Design review of the part built by this model. Coordinates are the model's own, in mm. Face numbers are marked on the shaded views. Coordinates: 2 decimals unless noted, no trailing zeros. Order: outer loops, then holes, each group sorted by start corner. A loop starts at its lowest first (then second) coordinate and runs counter-clockwise, first axis right, second up. Notation, with made-up numbers: M 86,56.5 L 135,56.5 A24 ccw 135,76.5 Z; hole C 1,6 d6. An arc over 180 degrees is marked long. Use CSV: the item, a comma, the result in double quotes.
```python
from build123d import *

# Parameters (mm, degrees)
SKETCH_3_R               = 40
EXTRUDE_2_DEPTH          = 5
CUT_EXTRUDE_2_DEPTH      = 10
SKETCH_6_R               = 2
CUT_EXTRUDE_3_DEPTH      = 10
SKETCH_8_R               = 3.5
SKETCH_8_R_2             = 2.5
EXTRUDE_3_DEPTH          = 8
PATTERN_CIRCULAR_1_COUNT = 3


with BuildPart() as part:
    # 草图3 → 凸台-拉伸2 (new body)
    with BuildSketch(Plane(origin=(0, 0, 0), x_dir=(1, 0, 0), z_dir=(0, 1, 0))):
        with Locations(Location((0, 0, 0), (0, 0, 270))):
            Circle(SKETCH_3_R)
    extrude(amount=EXTRUDE_2_DEPTH)

    # 草图5 → 切除-拉伸2 (cut)
    with BuildSketch(Plane(origin=(0, 5, 0), x_dir=(1, 0, 0), z_dir=(0, 1, 0))):
        with BuildLine():
            Line((-3, -29.849623113), (-3, 29.849623113))
            ThreePointArc((-3, 29.849623113), (-30, 0), (-3, -29.849623113))
        make_face()
        with BuildLine():
            ThreePointArc((30, 0), (22.248595461, 20.124611797), (3, 29.849623113))
            Line((3, 29.849623113), (3, -29.849623113))
            ThreePointArc((3, -29.849623113), (22.248595461, -20.124611797), (30, 0))
        make_face()
    extrude(amount=-CUT_EXTRUDE_2_DEPTH, mode=Mode.SUBTRACT)

    # 草图6 → 切除-拉伸3 (cut)
    with BuildSketch(Plane(origin=(0, 5, 0), x_dir=(1, 0, 0), z_dir=(0, 1, 0))):
        with Locations(Location((0, 0, 0), (0, 0, 270))):
            Circle(SKETCH_6_R)
    extrude(amount=-CUT_EXTRUDE_3_DEPTH, mode=Mode.SUBTRACT)

    # 草图8 → 凸台-拉伸3 (add)
    with BuildSketch(Plane(origin=(0, 5, 0), x_dir=(1, 0, 0), z_dir=(0, 1, 0))):
        with Locations(Location((0, -35, 0), (0, 0, 270))):
            Circle(SKETCH_8_R)
        with Locations(Location((0, -35, 0), (0, 0, 270))):
            Circle(SKETCH_8_R_2, mode=Mode.SUBTRACT)
    extrude_3 = extrude(amount=EXTRUDE_3_DEPTH)

    # 阵列(圆周)1: 凸台-拉伸3 ×3 about axis
    pattern_circular_1_axis = Axis((0, 0, 0), (0, 1, 0))
    for i in range(1, PATTERN_CIRCULAR_1_COUNT):
        add(extrude_3.rotate(pattern_circular_1_axis, i * 360 / PATTERN_CIRCULAR_1_COUNT))


solid = part.part
```
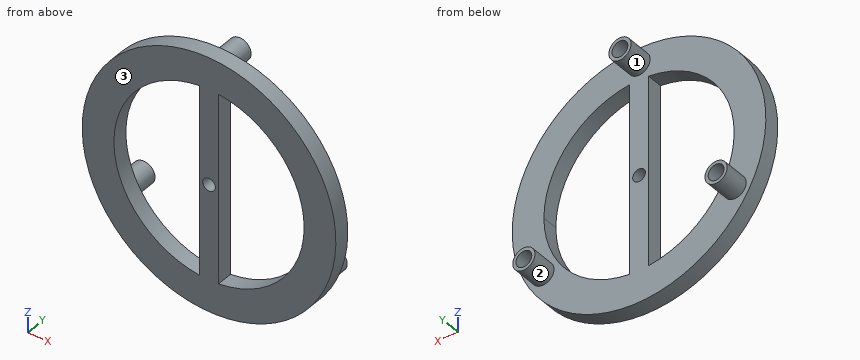
(1) Wall thickness on probe 1 along X at (y, z) = (1.65, 0); probe 2 along X at (y, z) = (11.25, -17.5); probe 3 along X at (y, z) = (3.5, -8.5): over which ranges is each line inside the solid? List them lowest first.
The answers:
probe 1,"x = -40 to -30, -3 to -2, 2 to 3, 30 to 40"
probe 2,"x = -33.81 to -32.81, -27.81 to -26.81, 26.81 to 27.81, 32.81 to 33.81"
probe 3,"x = -39.09 to -28.77, -3 to 3, 28.77 to 39.09"
(2) Clearance check with flat-ended pins moving along their axes: P1, Ø2.5, axis at y = 1.5, z = -9, coming from the +X side; P2, Ø2, axis at y = 4.5, z = -27.5, coming from the +X side; P3, Ø2.5, axis at x = -30, z = -18.5, coming from the +Y side; P4, Ø1.5, axis at x = 25, y = 6, coming from the -Z side. State where each tip first meets the part, or that it passes through.
The answers:
P1,"stops at x = 39.24"
P2,"stops at x = 29.96"
P3,"stops at y = 5"
P4,"passes through"
(3) Add section A-A on x = 0. State the section outline as (y, z) points, and give its area (3 significant figures).
The answers:
outline,"M 0,-40 L 5,-40 L 5,-2 L 0,-2 Z; M 0,2 L 5,2 L 5,31.5 L 13,31.5 L 13,32.5 L 5,32.5 L 5,37.5 L 13,37.5 L 13,38.5 L 5,38.5 L 5,40 L 0,40 Z"
area,"396 mm2"
(4) Add section D-D on y = 11.5. State the section outline as (x, z) points.
The answers:
outline,"C -30.31,-17.5 d7; C 0,35 d7; C 30.31,-17.5 d7; hole C -30.31,-17.5 d5; hole C 0,35 d5; hole C 30.31,-17.5 d5"
(5) Add section C-C on z = -3. State the section outline as (x, y) points, and give its area (3 significant figures).
The answers:
outline,"M -39.89,0 L -29.85,0 L -29.85,5 L -39.89,5 Z; M -3,0 L 3,0 L 3,5 L -3,5 Z; M 29.85,0 L 39.89,0 L 39.89,5 L 29.85,5 Z"
area,"130 mm2"
(6) The part is to be moulded in two halves that separate along X. For the marked faces 1, 2 and 3, say which applies: pulls with the +X half, pulls with the -X half, needs draft (parallel to the pull), parting line crosses it, or undercut.
The answers:
face 1,"parting line crosses it"
face 2,"undercut"
face 3,"needs draft"
(7) Add section B-B on y = 4. State the section outline as (x, z) points, and give its area (3 significant figures).
The answers:
outline,"C 0,0 d80; hole M -3,-29.85 L -3,29.85 A30 ccw Z; hole C 0,0 d4; hole M 3,-29.85 A30 ccw 3,29.85 Z"
area,"2,550 mm2"
